```python
from build123d import *

# Parameters (mm, degrees)
F0_R         = 2.54
F1_DEPTH     = 25.4
F2_R         = 2.5365962647
F3_DEPTH     = 60.706
F4_R         = 18.8716899986
F5_DEPTH     = 14.478
F6_DEPTH     = 1.778
F7_T1_DEPTH  = 46.7340686292
F7_T3_DEPTH  = 46.7340686292
F7_T5_DEPTH  = 9.4612519522
F7_S9_W      = 2.2367022539
F7_S9_H      = 2.2367022539
F7_T10_DEPTH = 2.236702254
F7_S15_W     = 2.2367022539
F7_S15_H     = 2.2367022539
F7_T16_DEPTH = 2.236702254
F7_S21_W     = 2.2367022539
F7_S21_H     = 2.2367022539
F7_T22_DEPTH = 2.236702254
F7_S27_W     = 2.2367022539
F7_S27_H     = 2.2367022539
F7_T28_DEPTH = 2.236702254


# Not quite as in the source:
# - a fillet or chamfer that OpenCascade refuses, or shapes differently, is made with other operations: its cross-section is extruded or revolved along the edge and cut away or added


with BuildPart() as f1:
    # F0 (on Front) → F1 (new body, symmetric)
    with BuildSketch(Plane.XZ):
        with BuildLine():
            Line((25.4, 14.5918969065), (25.4, 21.0037002322))
            ThreePointArc((25.4, 21.0037002322), (0, 23.2693725585), (-25.4, 21.0037002322))
            Line((-25.4, 21.0037002322), (-25.4, 14.5918969065))
            Line((-25.4, 14.5918969065), (25.4, 14.5918969065))
        make_face()
        with Locations((0, 18.9952347428)):
            Circle(F0_R, mode=Mode.SUBTRACT)
    extrude(amount=F1_DEPTH, both=True)

    # F2 (on face) → F3 (cut)
    with BuildSketch(Plane.YZ.offset(25.4)):
        with Locations((0, 17.843645066)):
            Circle(F2_R)
    extrude(amount=-F3_DEPTH, mode=Mode.SUBTRACT)

    # F4 (on face) → F5 (cut)
    with BuildSketch(Plane(origin=(0, 0, 14.5918969065), x_dir=(1, 0, 0), z_dir=(0, 0, -1))):
        Circle(F4_R)
    extrude(amount=-F5_DEPTH, mode=Mode.SUBTRACT)

    # F4 (on face) → F6 (join)
    with BuildSketch(Plane(origin=(0, 0, 14.5918969065), x_dir=(1, 0, 0), z_dir=(0, 0, -1))):
        Circle(F4_R)
    extrude(amount=-F6_DEPTH)

    # F7: fillet of radius 2.032 on 12 edges, made by hand

    # F7_s2 → F7_t1 (cut)
    with BuildSketch(Plane.XZ.offset(-23.3670343146)):
        with BuildLine():
            ThreePointArc((-25.4004, 16.6248625919), (-24.8048409794, 15.1870559271), (-23.3670343146, 14.5914969065))
            Line((-23.3670343146, 14.5914969065), (-23.3670343146, 14.388160338))
            ThreePointArc((-23.3670343146, 14.388160338), (-24.3835171573, 14.388560338), (-25.4, 14.388560338))
            Line((-25.4, 14.388560338), (-25.6033365685, 14.5918969065))
            ThreePointArc((-25.6033365685, 14.5918969065), (-25.6033365685, 15.6083797492), (-25.6037365685, 16.6248625919))
            Line((-25.6037365685, 16.6248625919), (-25.4004, 16.6248625919))
        make_face()
        with BuildLine():
            ThreePointArc((25.4004, 16.6248625919), (24.8048409794, 15.1870559271), (23.3670343146, 14.5914969065))
            Line((23.3670343146, 14.5914969065), (23.3670343146, 14.388160338))
            ThreePointArc((23.3670343146, 14.388160338), (24.3835171573, 14.388560338), (25.4, 14.388560338))
            Line((25.4, 14.388560338), (25.6033365685, 14.5918969065))
            ThreePointArc((25.6033365685, 14.5918969065), (25.6033365685, 15.6083797492), (25.6037365685, 16.6248625919))
            Line((25.6037365685, 16.6248625919), (25.4004, 16.6248625919))
        make_face()
    extrude(amount=F7_T1_DEPTH, mode=Mode.SUBTRACT)

    # F7_s4 → F7_t3 (cut)
    with BuildSketch(Plane.YZ.offset(-23.3670343146)):
        with BuildLine():
            ThreePointArc((23.3670343146, 14.5914969065), (24.8048409794, 15.1870559271), (25.4004, 16.6248625919))
            Line((25.4004, 16.6248625919), (25.6037365685, 16.6248625919))
            ThreePointArc((25.6037365685, 16.6248625919), (25.6033365685, 15.6083797492), (25.6033365685, 14.5918969065))
            Line((25.6033365685, 14.5918969065), (25.4, 14.388560338))
            ThreePointArc((25.4, 14.388560338), (24.3835171573, 14.388560338), (23.3670343146, 14.388160338))
            Line((23.3670343146, 14.388160338), (23.3670343146, 14.5914969065))
        make_face()
        with BuildLine():
            ThreePointArc((-25.4004, 16.6248625919), (-24.8048409794, 15.1870559271), (-23.3670343146, 14.5914969065))
            Line((-23.3670343146, 14.5914969065), (-23.3670343146, 14.388160338))
            ThreePointArc((-23.3670343146, 14.388160338), (-24.3835171573, 14.388560338), (-25.4, 14.388560338))
            Line((-25.4, 14.388560338), (-25.6033365685, 14.5918969065))
            ThreePointArc((-25.6033365685, 14.5918969065), (-25.6033365685, 15.6083797492), (-25.6037365685, 16.6248625919))
            Line((-25.6037365685, 16.6248625919), (-25.4004, 16.6248625919))
        make_face()
    extrude(amount=F7_T3_DEPTH, mode=Mode.SUBTRACT)

    # F7_s6 → F7_t5 (cut)
    with BuildSketch(Plane.XY.offset(16.6248625919)):
        with BuildLine():
            ThreePointArc((-25.4004, 23.3670343146), (-24.8048409794, 24.8048409794), (-23.3670343146, 25.4004))
            Line((-23.3670343146, 25.4004), (-23.3670343146, 25.6037365685))
            ThreePointArc((-23.3670343146, 25.6037365685), (-24.3835171573, 25.6033365685), (-25.4, 25.6033365685))
            Line((-25.4, 25.6033365685), (-25.6033365685, 25.4))
            ThreePointArc((-25.6033365685, 25.4), (-25.6033365685, 24.3835171573), (-25.6037365685, 23.3670343146))
            Line((-25.6037365685, 23.3670343146), (-25.4004, 23.3670343146))
        make_face()
        with BuildLine():
            ThreePointArc((-25.4004, -23.3670343146), (-24.8048409794, -24.8048409794), (-23.3670343146, -25.4004))
            Line((-23.3670343146, -25.4004), (-23.3670343146, -25.6037365685))
            ThreePointArc((-23.3670343146, -25.6037365685), (-24.3835171573, -25.6033365685), (-25.4, -25.6033365685))
            Line((-25.4, -25.6033365685), (-25.6033365685, -25.4))
            ThreePointArc((-25.6033365685, -25.4), (-25.6033365685, -24.3835171573), (-25.6037365685, -23.3670343146))
            Line((-25.6037365685, -23.3670343146), (-25.4004, -23.3670343146))
        make_face()
        with BuildLine():
            ThreePointArc((25.4004, -23.3670343146), (24.8048409794, -24.8048409794), (23.3670343146, -25.4004))
            Line((23.3670343146, -25.4004), (23.3670343146, -25.6037365685))
            ThreePointArc((23.3670343146, -25.6037365685), (24.3835171573, -25.6033365685), (25.4, -25.6033365685))
            Line((25.4, -25.6033365685), (25.6033365685, -25.4))
            ThreePointArc((25.6033365685, -25.4), (25.6033365685, -24.3835171573), (25.6037365685, -23.3670343146))
            Line((25.6037365685, -23.3670343146), (25.4004, -23.3670343146))
        make_face()
        with BuildLine():
            ThreePointArc((25.4004, 23.3670343146), (24.8048409794, 24.8048409794), (23.3670343146, 25.4004))
            Line((23.3670343146, 25.4004), (23.3670343146, 25.6037365685))
            ThreePointArc((23.3670343146, 25.6037365685), (24.3835171573, 25.6033365685), (25.4, 25.6033365685))
            Line((25.4, 25.6033365685), (25.6033365685, 25.4))
            ThreePointArc((25.6033365685, 25.4), (25.6033365685, 24.3835171573), (25.6037365685, 23.3670343146))
            Line((25.6037365685, 23.3670343146), (25.4004, 23.3670343146))
        make_face()
    extrude(amount=F7_T5_DEPTH, mode=Mode.SUBTRACT)


with BuildPart() as f7_tool8:
    # F7_s9 → F7_t10 (new body)
    with BuildSketch(Plane.YZ.offset(-23.3670343146)):
        with Locations((24.4853854416, 15.506511465)):
            Rectangle(F7_S9_W, F7_S9_H)
    extrude(amount=-F7_T10_DEPTH)

    # F7_s11 → F7_t12 (revolve, cut)
    with BuildSketch(Plane(origin=(-23.3670343146, 23.3670343146, 16.6248625919), x_dir=(0, -0.7071067812, 0.7071067812), z_dir=(0, -0.7071067812, -0.7071067812))):
        with BuildLine():
            ThreePointArc((0, -2.0333656854), (2.0333656854, 0), (0, 2.0333656854))
            Line((0, 2.0333656854), (0, -2.0333656854))
        make_face()
    revolve(axis=Axis((-23.3670343146, 23.3670343146, 16.6248625919), (-1, 0, 0)), mode=Mode.SUBTRACT)


with BuildPart() as f1_1:
    add(f1.part)

    # F7_t7: cut F7_tool8
    add(f7_tool8.part, mode=Mode.SUBTRACT)


with BuildPart() as f7_tool14:
    # F7_s15 → F7_t16 (new body)
    with BuildSketch(Plane.YZ.offset(-23.3670343146)):
        with Locations((-24.4853854416, 15.506511465)):
            Rectangle(F7_S15_W, F7_S15_H)
    extrude(amount=-F7_T16_DEPTH)

    # F7_s17 → F7_t18 (revolve, cut)
    with BuildSketch(Plane(origin=(-23.3670343146, -23.3670343146, 16.6248625919), x_dir=(0, 0.7071067812, 0.7071067812), z_dir=(0, -0.7071067812, 0.7071067812))):
        with BuildLine():
            ThreePointArc((0, -2.0333656854), (2.0333656854, 0), (0, 2.0333656854))
            Line((0, 2.0333656854), (0, -2.0333656854))
        make_face()
    revolve(axis=Axis((-23.3670343146, -23.3670343146, 16.6248625919), (-1, 0, 0)), mode=Mode.SUBTRACT)


with BuildPart() as f1_2:
    add(f1_1.part)

    # F7_t13: cut F7_tool14
    add(f7_tool14.part, mode=Mode.SUBTRACT)


with BuildPart() as f7_tool20:
    # F7_s21 → F7_t22 (new body)
    with BuildSketch(Plane.XY.offset(16.6248625919)):
        with Locations((24.4853854416, 24.4853854416)):
            Rectangle(F7_S21_W, F7_S21_H)
    extrude(amount=-F7_T22_DEPTH)

    # F7_s23 → F7_t24 (revolve, cut)
    with BuildSketch(Plane(origin=(23.3670343146, 23.3670343146, 16.6248625919), x_dir=(-0.7071067812, -0.7071067812, 0), z_dir=(0.7071067812, -0.7071067812, 0))):
        with BuildLine():
            ThreePointArc((0, -2.0333656854), (2.0333656854, 0), (0, 2.0333656854))
            Line((0, 2.0333656854), (0, -2.0333656854))
        make_face()
    revolve(axis=Axis((23.3670343146, 23.3670343146, 16.6248625919), (0, 0, -1)), mode=Mode.SUBTRACT)


with BuildPart() as f1_3:
    add(f1_2.part)

    # F7_t19: cut F7_tool20
    add(f7_tool20.part, mode=Mode.SUBTRACT)


with BuildPart() as f7_tool26:
    # F7_s27 → F7_t28 (new body)
    with BuildSketch(Plane.XZ.offset(23.3670343146)):
        with Locations((24.4853854416, 15.506511465)):
            Rectangle(F7_S27_W, F7_S27_H)
    extrude(amount=F7_T28_DEPTH)

    # F7_s29 → F7_t30 (revolve, cut)
    with BuildSketch(Plane(origin=(23.3670343146, -23.3670343146, 16.6248625919), x_dir=(-0.7071067812, 0, 0.7071067812), z_dir=(0.7071067812, 0, 0.7071067812))):
        with BuildLine():
            ThreePointArc((0, -2.0333656854), (2.0333656854, 0), (0, 2.0333656854))
            Line((0, 2.0333656854), (0, -2.0333656854))
        make_face()
    revolve(axis=Axis((23.3670343146, -23.3670343146, 16.6248625919), (0, -1, 0)), mode=Mode.SUBTRACT)


with BuildPart() as f1_4:
    add(f1_3.part)

    # F7_t25: cut F7_tool26
    add(f7_tool26.part, mode=Mode.SUBTRACT)

    # F7_s31 → F7_t32 (revolve, cut)
    with BuildSketch(Plane.XY.offset(18.9952347428)):
        with BuildLine():
            ThreePointArc((2.5396, 23.3670343146), (3.1351590206, 24.8048409794), (4.5729656854, 25.4004))
            Line((4.5729656854, 25.4004), (4.5729656854, 25.6037365685))
            ThreePointArc((4.5729656854, 25.6037365685), (3.5564828427, 25.6033365685), (2.54, 25.6033365685))
            Line((2.54, 25.6033365685), (2.3366634315, 25.4))
            ThreePointArc((2.3366634315, 25.4), (2.3366634315, 24.3835171573), (2.3362634315, 23.3670343146))
            Line((2.3362634315, 23.3670343146), (2.5396, 23.3670343146))
        make_face()
    revolve(axis=Axis((0, 25.4, 18.9952347428), (0, -1, 0)), mode=Mode.SUBTRACT)

    # F7_s33 → F7_t34 (revolve, cut)
    with BuildSketch(Plane.XY.offset(17.843645066)):
        with BuildLine():
            ThreePointArc((23.3670343146, 2.5361962647), (24.8048409794, 3.1317552853), (25.4004, 4.5695619501))
            Line((25.4004, 4.5695619501), (25.6037365685, 4.5695619501))
            ThreePointArc((25.6037365685, 4.5695619501), (25.6033365685, 3.5530791074), (25.6033365685, 2.5365962647))
            Line((25.6033365685, 2.5365962647), (25.4, 2.3332596961))
            ThreePointArc((25.4, 2.3332596961), (24.3835171573, 2.3332596961), (23.3670343146, 2.3328596961))
            Line((23.3670343146, 2.3328596961), (23.3670343146, 2.5361962647))
        make_face()
    revolve(axis=Axis((25.4, 0, 17.843645066), (1, 0, 0)), mode=Mode.SUBTRACT)

    # F7_s35 → F7_t36 (revolve, cut)
    with BuildSketch(Plane.XY.offset(18.9952347428)):
        with BuildLine():
            ThreePointArc((2.5396, -23.3670343146), (3.1351590206, -24.8048409794), (4.5729656854, -25.4004))
            Line((4.5729656854, -25.4004), (4.5729656854, -25.6037365685))
            ThreePointArc((4.5729656854, -25.6037365685), (3.5564828427, -25.6033365685), (2.54, -25.6033365685))
            Line((2.54, -25.6033365685), (2.3366634315, -25.4))
            ThreePointArc((2.3366634315, -25.4), (2.3366634315, -24.3835171573), (2.3362634315, -23.3670343146))
            Line((2.3362634315, -23.3670343146), (2.5396, -23.3670343146))
        make_face()
    revolve(axis=Axis((0, -25.4, 18.9952347428), (0, -1, 0)), mode=Mode.SUBTRACT)

    # F7_s37 → F7_t38 (revolve, cut)
    with BuildSketch(Plane.XY.offset(17.843645066)):
        with BuildLine():
            ThreePointArc((-25.4004, 4.5695619501), (-24.8048409794, 3.1317552853), (-23.3670343146, 2.5361962647))
            Line((-23.3670343146, 2.5361962647), (-23.3670343146, 2.3328596961))
            ThreePointArc((-23.3670343146, 2.3328596961), (-24.3835171573, 2.3332596961), (-25.4, 2.3332596961))
            Line((-25.4, 2.3332596961), (-25.6033365685, 2.5365962647))
            ThreePointArc((-25.6033365685, 2.5365962647), (-25.6033365685, 3.5530791074), (-25.6037365685, 4.5695619501))
            Line((-25.6037365685, 4.5695619501), (-25.4004, 4.5695619501))
        make_face()
    revolve(axis=Axis((-25.4, 0, 17.843645066), (1, 0, 0)), mode=Mode.SUBTRACT)


solid = f1_4.part
```
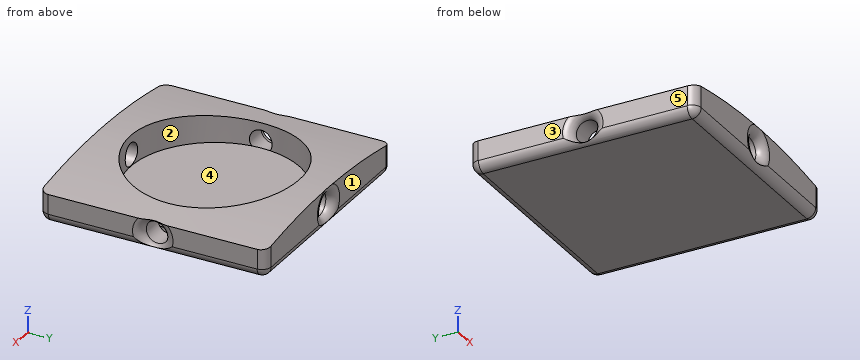
Geometry check sheet. Reference: the model listing, model coordinates, mm. Face numbers are marked on the shaded views. A direction names the side the tool comes from. Coordinates: 2 decimals unless noted, no trailing zeros. Write each loop counter-clockwise with the first axis right and the second up, starting at its lowest first coordinate (ties: lowest second). Pieces come first, ordered by that corner, then holes. Notation, with made-up numbers: M -36.5,82.25 L 5.5,82.25 A26 cw 5.5,108.25 Z; hole C 85,26.5 d6. An arc over 180 degrees is marked long. Use one line per item in the form item = value. Start each with the question number.
1) Section check D-D on y = 21. Enter the section's corners in (x, z).
2) Section check A-A on x = 0. Enter the section's corners in (y, z).
3) Thickness scan on probe 1 along Z at (x, y) = (0, -19); probe 2 along Y at (x, z) = (-13.5, 18.25); probe 3 along X at (y, z) = (-11.5, 17.5). Record the ranges inside material, lowest first. Write a range as from..to.
4) Section check B-B on y = 0. Enter the section's corners in (x, z).
5) Set-up check for the marked faces 4 and 5: record each of +Z, -Z, +X, -X, +Y, -Y from which the full face is reachable in a straight line by a thin tool's end or side.
6) Go/stop test with flat-tipped pins: pin 1 Ø3 at (x, y) = (11.5, -15) entering from +Z; pin 2 Ø19 at (x, y) = (-5, -2) entering from +Z; pin 3 Ø1 at (x, z) = (3, 17.5) entering from +Y; pin 4 Ø4.5 at (x, z) = (0, 19) entering from +Y. Record where each tip stops, or that it passes through.
7) Release check for a two-part mould opening along Y. For the marked faces 1, 2 and 3 record: pulls with the +Y half, pulls with the -Y half, needs draft (parallel to the pull), parting line crosses it, or undercut.
8) Section check C-C on x = -6.5. Enter the section's corners in (y, z), and give its area (3 significant figures).
Responses:
q1.outline = M -25.4,16.58 A2.03 ccw -23.41,14.59 L 23.41,14.59 A2.03 ccw 25.4,16.58 L 25.4,21 A143.51 ccw -25.4,21 Z; hole C 0,19 d5.08
q2.outline = M -25.38,23.27 A2.03 ccw -23.41,21.54 L -18.87,21.54 L -18.87,23.27 Z; M -25.08,15.52 A2.03 ccw -23.41,14.59 L 23.41,14.59 A2.03 ccw 25.08,15.52 A2.03 ccw 23.41,16.46 L 18.87,16.46 L 18.87,16.37 L -18.87,16.37 L -18.87,16.46 L -23.41,16.46 A2.03 ccw Z; M 18.87,21.54 L 23.41,21.54 A2.03 ccw 25.38,23.27 L 18.87,23.27 Z
q3.probe_1 = 14.59..16.46, 21.54..23.27
q3.probe_2 = -25.4..-13.19, 13.19..25.4
q3.probe_3 = -25.4..-14.96, 14.96..25.4
q4.outline = M -24.91,21.09 A2.03 ccw -23.41,20.38 L -18.87,20.38 L -18.87,22.02 A143.51 ccw Z; M -24.52,14.95 A2.03 ccw -23.41,14.59 L 23.41,14.59 A2.03 ccw 24.52,14.95 A2.03 ccw 23.41,15.31 L 18.87,15.31 L 18.87,16.37 L -18.87,16.37 L -18.87,15.31 L -23.41,15.31 A2.03 ccw Z; M 18.87,20.38 L 23.41,20.38 A2.03 ccw 24.91,21.09 A143.51 ccw 18.87,22.02 Z
q5.face_4 = +Z
q5.face_5 = +Z, -Z, -X, +Y, -Y
q6.pin_1 = 22.9
q6.pin_2 = 16.37
q6.pin_3 = 25.27
q6.pin_4 = through
q7.face_1 = pulls with the +Y half
q7.face_2 = undercut
q7.face_3 = needs draft
q8.outline = M -25.4,16.58 A2.03 ccw -23.41,14.59 L 23.41,14.59 A2.03 ccw 25.4,16.58 L 25.4,23.12 L 17.72,23.12 L 17.72,16.37 L -17.72,16.37 L -17.72,23.12 L -25.4,23.12 Z
q8.area = 192 mm2
